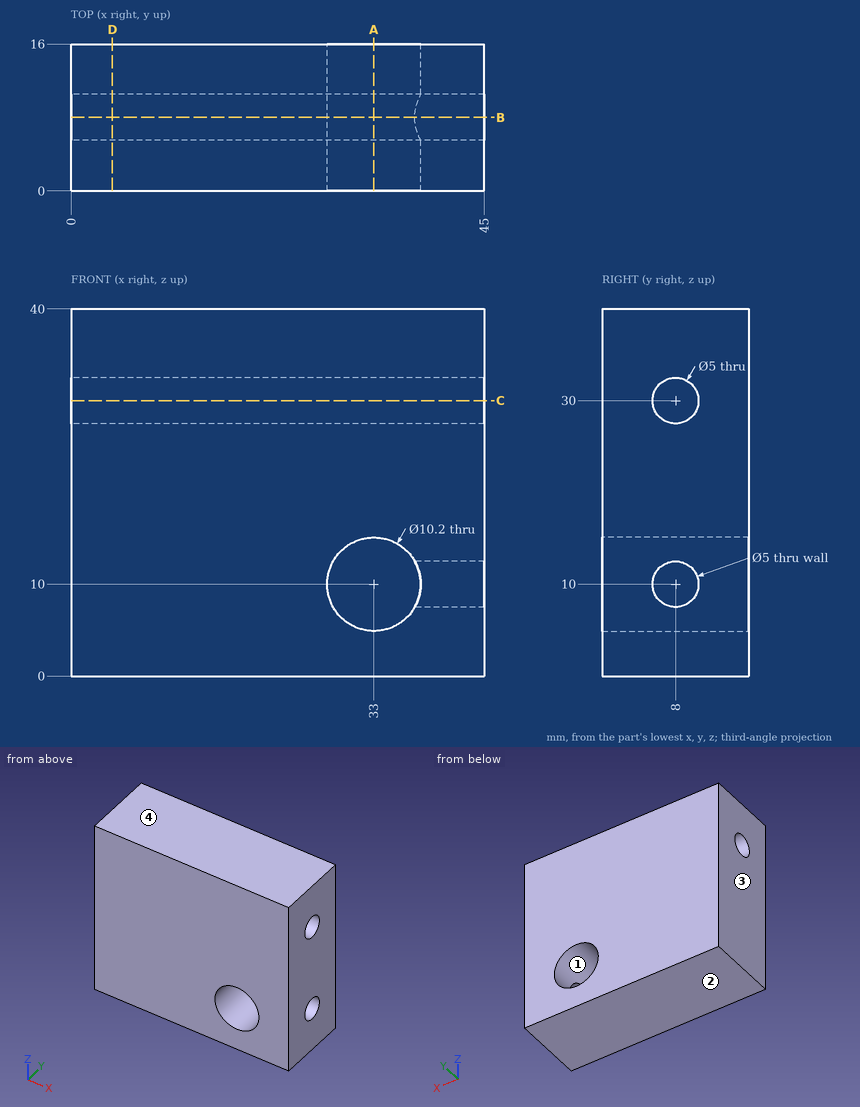
Source: three-view drawing plus pictorial views. Frame: mm from the lowest corner of the part. Round coordinates to 2 decimals unless told otherwise and drop trailing zeros. Loops run counter-clockwise (first coordinate to the right, second up) from the corner with the lowest first, then second, coordinate; pieces in that order, holes last. Notation, with made-up numbers: (-20.75, 80.25) -> (-1.75, 80.25) arc R19 ccw to (-1.75, 89.25) -> close; hole circle Ø2 at (5, 37.5). An arc over 180 degrees is marked (long way). Use one line per item in the form item = value.
Item 1: Draft query along Z for the marked faces 1, 2, 3 and 4. Return one class per face: released by +Z, released by -Z, zero draft, split by the parting line, or undercut.
Evaluation:
face_1 = undercut
face_2 = released by -Z
face_3 = zero draft
face_4 = released by +Z
Item 2: Material intervals for probe 1 along X at (y, z) = (11.75, 10); probe 2 along Z at (x, y) = (3.5, 8.25); probe 3 along Y at (x, z) = (35, 30), sorted ascending.
Evaluation:
probe_1 = 0 to 27.9, 38.1 to 45
probe_2 = 0 to 27.51, 32.49 to 40
probe_3 = 0 to 5.5, 10.5 to 16
Item 3: Cut plane B-B on y = 8. Output: boundary loops of the cut face in (x, z).
Evaluation:
outline = (0, 0) -> (45, 0) -> (45, 7.5) -> (37.45, 7.5) arc R5.1 cw (long way) to (37.45, 12.5) -> (45, 12.5) -> (45, 27.5) -> (0, 27.5) -> close; (0, 32.5) -> (45, 32.5) -> (45, 40) -> (0, 40) -> close
Item 4: Cut plane D-D on x = 4.5. Output: boundary loops of the cut face in (y, z).
Evaluation:
outline = (0, 0) -> (16, 0) -> (16, 40) -> (0, 40) -> close; hole circle Ø5 at (8, 30)
Item 5: Cut plane C-C on z = 30. Output: boundary loops of the cut face in (x, y).
Evaluation:
outline = (0, 0) -> (45, 0) -> (45, 5.5) -> (0, 5.5) -> close; (0, 10.5) -> (45, 10.5) -> (45, 16) -> (0, 16) -> close
Item 6: Cut plane A-A on x = 33. Output: boundary loops of the cut face in (y, z), then the cut area to 3 significant figures.
Evaluation:
outline = (0, 0) -> (16, 0) -> (16, 4.9) -> (0, 4.9) -> close; (0, 15.1) -> (16, 15.1) -> (16, 40) -> (0, 40) -> close; hole circle Ø5 at (8, 30)
area = 457 mm2
